For this review, take the finished solid that the model builds, in its own axes (mm). A direction names the side the tool comes from. Coordinates: 2 decimals unless noted, no trailing zeros. Loops run counter-clockwise (first coordinate to the right, second up) from the corner with the lowest first, then second, coordinate; pieces in that order, holes last. Notation, with made-up numbers: (38, 43) -> (76, 43) arc R11 cw to (76, 55) -> close; hole circle Ø7 at (-18.75, -1). An arc over 180 degrees is marked (long way). One line per item, written item: value.
from build123d import *

# Parameters (mm, degrees)
F1_DEPTH       = 30
F3_D           = 8
F3_DEPTH       = 45
F3_CBORE_D     = 14
F3_CBORE_DEPTH = 9
F5_R           = 21
F6_DEPTH       = 25


with BuildPart() as f1:
    # F0 (on Front) → F1 (new body)
    with BuildSketch(Plane.XZ):
        Polygon((87, 0), (0, 0), (0, -124), (124, -124), (124, -27), (106, -14.071459), (100, -14), align=None)
    extrude(amount=F1_DEPTH)

    # F3
    with Locations(Plane.XZ.offset(30)):
        with Locations((15, -23), (10, -92), (112, -32), (114, -105)):
            CounterBoreHole(F3_D / 2, F3_CBORE_D / 2, F3_CBORE_DEPTH, depth=F3_DEPTH)

    # F5 (on face) → F6 (cut)
    with BuildSketch(Plane(origin=(0, 0, 0), x_dir=(-1, 0, 0), z_dir=(0, 1, 0))):
        with Locations((-61.409097, -64.425051)):
            Circle(F5_R)
    extrude(amount=-F6_DEPTH, mode=Mode.SUBTRACT)


solid = f1.part
1. Take a section at C-C, the plane x = 112. Give the boundary of the cut face in (y, z).
Return value:
outline: (-30, -124) -> (0, -124) -> (0, -108.46) -> (-21, -108.46) -> (-21, -111.71) -> (-30, -111.71) -> close; (-30, -98.29) -> (-21, -98.29) -> (-21, -101.54) -> (0, -101.54) -> (0, -36) -> (-21, -36) -> (-21, -39) -> (-30, -39) -> close; (-30, -25) -> (-21, -25) -> (-21, -28) -> (0, -28) -> (0, -18.38) -> (-30, -18.38) -> close
2. The part is to be moulded in two halves that separate along Z. For faces 1 (the flat face through (44, -15, 0)), 2 (the flat face through (117, -21, -108)), 3 (the flat face through (0, -15, -61)), say which applies: pulls with the +Z half, pulls with the -Z half, needs draft (parallel to the pull), parting line crosses it, or undercut.
Return value:
face 1: pulls with the +Z half
face 2: undercut
face 3: needs draft
3. Insertion check: pin 1 Ø13 at (x, z) = (112, -32) entering from -Y; pin 2 Ø21 at (x, z) = (62, -56.5) entering from +Y. Each pin has a flat end and moves straight along its axis. Give the tip position at first contact, or say it passes through.
Return value:
pin 1: stops at y = -21
pin 2: stops at y = -25
4. Take a section at A-A, the plane z = -32. Give the boundary of the cut face in (x, y).
Return value:
outline: (0, -30) -> (105, -30) -> (105, -21) -> (108, -21) -> (108, 0) -> (0, 0) -> close; (116, -21) -> (119, -21) -> (119, -30) -> (124, -30) -> (124, 0) -> (116, 0) -> close
5. For faces 4 (the flat face through (93.591, -14.79, -7.098)), 5 (the cylindrical face through (51.719, -12.325, -83.056)), 6 (the flat face through (13, -21, -95)), list the 3-axis set-ups (+Z, -Z, +X, -X, +Y, -Y) from which the entire face can be reached by the end or side of a thin tool; tool diameter is ignored.
Return value:
face 4: +Z, +X, +Y, -Y
face 5: +Y
face 6: -Y
6. Take a section at B-B, the plane y = -27.5. Give the boundary of the cut face in (x, z), and give its area (3 significant figures).
Return value:
outline: (0, -124) -> (124, -124) -> (124, -27) -> (106, -14.07) -> (100, -14) -> (87, 0) -> (0, 0) -> close; hole circle Ø14 at (10, -92); hole circle Ø14 at (15, -23); hole circle Ø14 at (112, -32); hole circle Ø14 at (114, -105)
area: 14,200 mm2
7. To check wall thickness, follow probe 1 along Z at (x, y) = (111, -16.75); probe 2 along Z at (x, y) = (112, -5.5); probe 3 along Z at (x, y) = (10, -11). State the ranges of each line that lie inside material, in increasing order. Write a range as from..to.
Return value:
probe 1: z = -124..-107.65, -102.35..-35.87, -28.13..-17.66
probe 2: z = -124..-108.46, -101.54..-36, -28..-18.38
probe 3: z = -124..-96, -88..0
8. Take a section at D-D, the plane y = -16. Give the boundary of the cut face in (x, z).
Return value:
outline: (0, -124) -> (124, -124) -> (124, -27) -> (106, -14.07) -> (100, -14) -> (87, 0) -> (0, 0) -> close; hole circle Ø8 at (10, -92); hole circle Ø8 at (15, -23); hole circle Ø42 at (61.41, -64.43); hole circle Ø8 at (112, -32); hole circle Ø8 at (114, -105)
